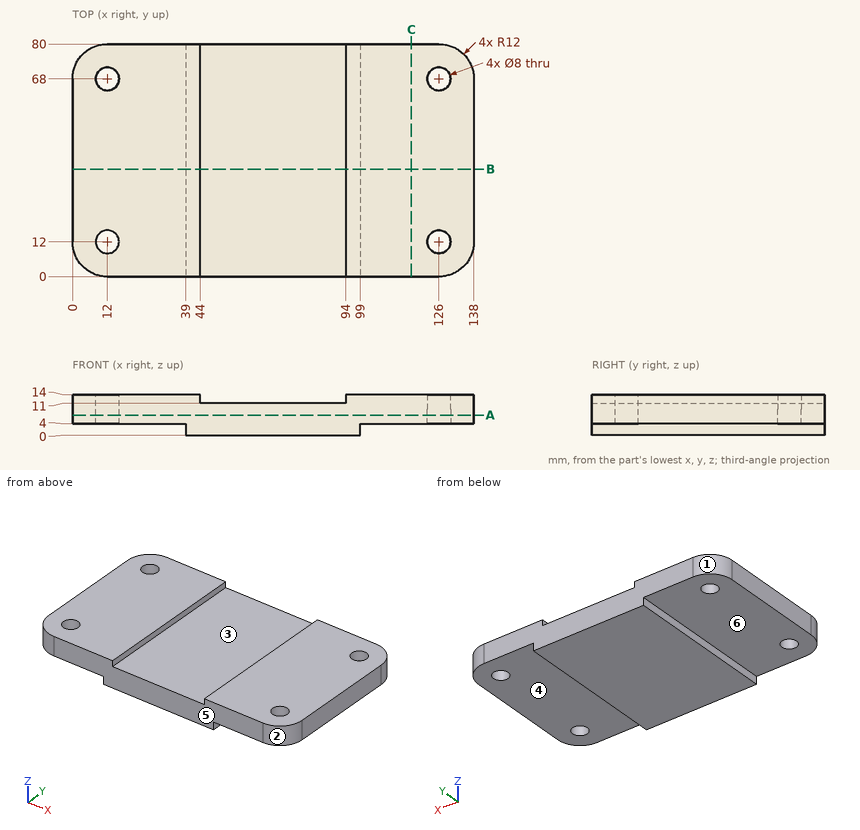
Source: three-view drawing plus pictorial views. Frame: mm from the lowest corner of the part. A direction names the side the tool comes from. Give positions to 0.01 mm unless a question says otherwise; leave off trailing zeros. Order: outer loops, then holes, each group sorted by start corner. A loop starts at its lowest first (then second) coordinate and runs counter-clockwise, first axis right, second up.
1. Mould query, pull axis X, two halves, no side actions, for the marked faces 1, 2 and 3. Classes: released by +X, released by -X, zero draft, split by the parting line, or undercut.
Derived:
face 1: released by -X
face 2: released by +X
face 3: undercut
2. Section A-A on z = 7. Return the cut outline in (x, y), and give its area (3 significant figures).
Derived:
outline: (0, 12) arc R12 ccw to (12, 0) - (126, 0) arc R12 ccw to (138, 12) - (138, 68) arc R12 ccw to (126, 80) - (12, 80) arc R12 ccw to (0, 68) - close; hole circle Ø8 at (12, 12); hole circle Ø8 at (12, 68); hole circle Ø8 at (126, 12); hole circle Ø8 at (126, 68)
area: 10,700 mm2
3. Reachability of the marked faces 4, 5 and 6 from +Z, -Z, +X, -X, +Y, -Y: full face, straight path, thin tool, end or side. Return the list, or none.
Derived:
face 4: -Z, +X, +Y, -Y
face 5: +Z, -Z, +X, -X, -Y
face 6: -Z, -X, +Y, -Y
4. Material intervals for L1, parallel to Y at x = 126, z = 10.65; L2, parallel to X at y = 68, z = 12.75; L3, parallel to Y at x = 127.5, z = 12, sorted ascending.
Derived:
L1: y = 0 to 8, 16 to 64, 72 to 80
L2: x = 0 to 8, 16 to 44, 94 to 122, 130 to 138
L3: y = 0.09 to 8.29, 15.71 to 64.29, 71.71 to 79.91
5. Section B-B on y = 37. Return the cut outline in (x, z).
Derived:
outline: (0, 4) - (39, 4) - (39, 0) - (99, 0) - (99, 4) - (138, 4) - (138, 14) - (94, 14) - (94, 11) - (44, 11) - (44, 14) - (0, 14) - close
6. Pin query (flat end, axial travel): pin 1 (1.5 mm diameter, centred on x = 92.5, y = 65, fed in from +Z); pin 2 (5 mm diameter, centred on x = 12, y = 12, fed in from +Z); pin 3 (19.5 mm diameter, centred on x = 22, y = 42, fed in from -Z); pin 4 (3 mm diameter, centred on y = 34, z = 1.5, fed in from -X). Return the tip coordinate at first contact, or that it passes through.
Derived:
pin 1: stops at z = 11
pin 2: passes through
pin 3: stops at z = 4
pin 4: stops at x = 39
7. Section C-C on x = 116.5. Return the cut outline in (y, z), and give its area (3 significant figures).
Derived:
outline: (0, 4) - (80, 4) - (80, 14) - (0, 14) - close
area: 800 mm2
